from build123d import *

# Parameters (mm, degrees)
MODEL_R             = 1.6
BOSS_EXTRUDE1_DEPTH = 3.125


with BuildPart() as part:
    # Model → Boss-Extrude1 (new body)
    with BuildSketch(Plane.XY):
        with BuildLine():
            Line((194.5, 257.413429511), (102.5, 257.413429511))
            ThreePointArc((102.5, 257.413429511), (99.671572875, 256.241856636), (98.5, 253.413429511))
            Line((98.5, 253.413429511), (98.5, 242.617341429))
            ThreePointArc((98.5, 242.617341429), (33.751633999, 186.163429511), (17.235295135, 101.862743741))
            Line((17.235295135, 101.862743741), (7.885608595, 96.4646997))
            ThreePointArc((7.885608595, 96.4646997), (6.02190529, 94.035874265), (6.42150698, 91.000598085))
            Line((6.42150698, 91.000598085), (52.42150698, 11.326260937))
            ThreePointArc((52.42150698, 11.326260937), (54.850332414, 9.462557632), (57.885608595, 9.862159322))
            Line((57.885608595, 9.862159322), (67.235295135, 15.260203363))
            ThreePointArc((67.235295135, 15.260203363), (148.5, -12.586570489), (229.764704865, 15.260203363))
            Line((229.764704865, 15.260203363), (239.114391405, 9.862159322))
            ThreePointArc((239.114391405, 9.862159322), (242.149667586, 9.462557632), (244.57849302, 11.326260937))
            Line((244.57849302, 11.326260937), (290.57849302, 91.000598085))
            ThreePointArc((290.57849302, 91.000598085), (290.97809471, 94.035874265), (289.114391405, 96.4646997))
            Line((289.114391405, 96.4646997), (279.764704865, 101.862743741))
            ThreePointArc((279.764704865, 101.862743741), (263.248366001, 186.163429511), (198.5, 242.617341429))
            Line((198.5, 242.617341429), (198.5, 253.413429511))
            ThreePointArc((198.5, 253.413429511), (197.328427125, 256.241856636), (194.5, 257.413429511))
        make_face()
        with Locations((105.3, 249.913429511)):
            Circle(MODEL_R, mode=Mode.SUBTRACT)
        with Locations((191.7, 249.513429511)):
            Circle(MODEL_R, mode=Mode.SUBTRACT)
        with Locations((282.33689233, 92.525726954)):
            Circle(MODEL_R, mode=Mode.SUBTRACT)
        with Locations((239.13689233, 17.701132067)):
            Circle(MODEL_R, mode=Mode.SUBTRACT)
        with Locations((14.66310767, 92.525726954)):
            Circle(MODEL_R, mode=Mode.SUBTRACT)
        with Locations((57.86310767, 17.701132067)):
            Circle(MODEL_R, mode=Mode.SUBTRACT)
    extrude(amount=BOSS_EXTRUDE1_DEPTH)


solid = part.part
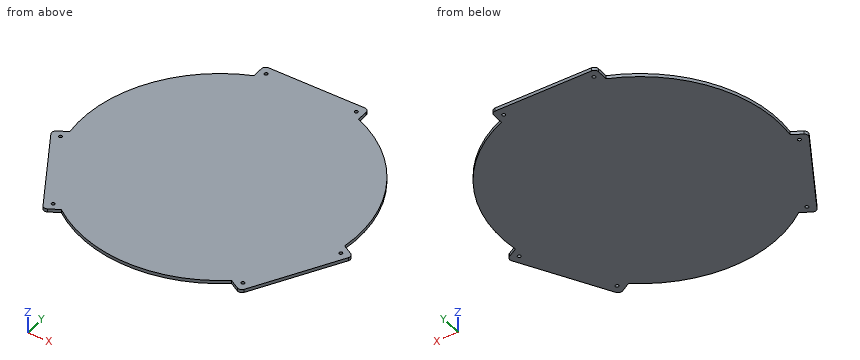
Here's how the part is built. I have some questions about the finished solid (model axes, mm). Give positions to 0.01 mm unless a question says otherwise; leave off trailing zeros. Loops run counter-clockwise (first coordinate to the right, second up) from the corner with the lowest first, then second, coordinate; pieces in that order, holes last. Notation, with made-up numbers: (-20, 32.25) -> (24, 32.25) arc R17 cw to (24, 63.25) -> close; hole circle Ø4 at (-2, 5.25). An arc over 180 degrees is marked (long way). Answer as a JSON object with one key per item and string values. Group by question number.
Item 1: I need wall thicknesses on L1, parallel to Y at x = 58, z = 0.4; L2, parallel to X at y = 111, z = 0.6; L3, parallel to Y at x = 105.3, z = 2.3. Which ranges of each line are inside material? Lowest first, please.
Item 2: Imagine slicing it at B-B on y = 76. Write out the boundary of the cut face in (x, z) (3 decimals).
Item 3: Imagine slicing it at C-C on y = 168.5. Write out the boundary of the cut face in (x, z) (3 decimals).
Item 4: Imagine slicing it at A-A on z = 0.7. Write out the boundary of the cut face in (x, y).
Item 5: Will these pins go through, and if not, where does the flat tip stop? pin 1 (1 mm diameter, centred on y = 20.5, z = 0.5, fed in from -X); pin 2 (1.6 mm diameter, centred on y = 247.5, z = 1.5, fed in from -X); pin 3 (1 mm diameter, centred on y = 67.5, z = 2, fed in from -X).
Answer list:
{
 "1": {"L1": "y = 9.93 to 16.11, 19.3 to 216.69", "L2": "x = 16.3 to 280.7", "L3": "y = -5.35 to 248.31, 251.51 to 257.41"},
 "2": {"outline": "(15.082, 0) -> (281.918, 0) -> (281.918, 3.125) -> (15.082, 3.125) -> close"},
 "3": {"outline": "(25.23, 0) -> (271.77, 0) -> (271.77, 3.125) -> (25.23, 3.125) -> close"},
 "4": {"outline": "(6.42, 91) -> (52.42, 11.33) arc R4 ccw to (57.89, 9.86) -> (67.24, 15.26) arc R132.5 ccw to (229.76, 15.26) -> (239.11, 9.86) arc R4 ccw to (244.58, 11.33) -> (290.58, 91) arc R4 ccw to (289.11, 96.46) -> (279.76, 101.86) arc R132.5 ccw to (198.5, 242.62) -> (198.5, 253.41) arc R4 ccw to (194.5, 257.41) -> (102.5, 257.41) arc R4 ccw to (98.5, 253.41) -> (98.5, 242.62) arc R132.5 ccw to (17.24, 101.86) -> (7.89, 96.46) arc R4 ccw to start; hole circle Ø3.2 at (14.66, 92.53); hole circle Ø3.2 at (57.86, 17.7); hole circle Ø3.2 at (105.3, 249.91); hole circle Ø3.2 at (191.7, 249.51); hole circle Ø3.2 at (239.14, 17.7); hole circle Ø3.2 at (282.34, 92.53)"},
 "5": {"pin 1": "stops at x = 46.84", "pin 2": "stops at x = 98.5", "pin 3": "stops at x = 19.7"}
}
